from build123d import *

# Parameters (mm, degrees)
SKETCH_1_R          = 3.5
EXTRUDE_1_DEPTH     = 3
SKETCH_2_R          = 2
EXTRUDE_2_DEPTH     = 1
SKETCH_3_R          = 1.5
EXTRUDE_3_DEPTH     = 8
SKETCH_4_R          = 1
CUT_EXTRUDE_1_DEPTH = 1.5
FILLET_1_R          = 0.5
CHAMFER_1_SIZE      = 0.5


with BuildPart() as part:
    # 草图1 → 凸台-拉伸1 (new body)
    with BuildSketch(Plane(origin=(0, 0, 0), x_dir=(1, 0, 0), z_dir=(0, 1, 0))):
        with Locations(Location((0, 0, 0), (0, 0, 270))):
            Circle(SKETCH_1_R)
    extrude(amount=EXTRUDE_1_DEPTH)

    # 草图2 → 凸台-拉伸2 (add)
    with BuildSketch(Plane(origin=(0, 3, 0), x_dir=(1, 0, 0), z_dir=(0, 1, 0))):
        with Locations(Location((0, 0, 0), (0, 0, 270))):
            Circle(SKETCH_2_R)
    extrude(amount=EXTRUDE_2_DEPTH)

    # 草图3 → 凸台-拉伸3 (add)
    with BuildSketch(Plane(origin=(0, 4, 0), x_dir=(1, 0, 0), z_dir=(0, 1, 0))):
        with Locations(Location((0, 0, 0), (0, 0, 270))):
            Circle(SKETCH_3_R)
    extrude(amount=EXTRUDE_3_DEPTH)

    # 草图4 → 切除-拉伸1 (cut)
    with BuildSketch(Plane.XZ):
        with Locations(Location((0, 0, 0), (0, 0, 270))):
            Circle(SKETCH_4_R)
    extrude(amount=-CUT_EXTRUDE_1_DEPTH, mode=Mode.SUBTRACT)

    # 圆角1
    fillet_1_edges = [part.edges().sort_by_distance(p)[0] for p in [
        (0, 0, -3.5),
        (0, 3, -3.5),
    ]]
    fillet(fillet_1_edges, radius=FILLET_1_R)

    # 倒角1
    chamfer_1_edges = [part.edges().sort_by_distance(p)[0] for p in [
        (0, 12, -1.5),
    ]]
    chamfer(chamfer_1_edges, length=CHAMFER_1_SIZE)


solid = part.part
Input: part model. Units: mm. Frame: model coordinates. A direction names the side the tool comes from. Round coordinates to 2 decimals unless told otherwise and drop trailing zeros. Order: outer loops, then holes, each group sorted by start corner. A loop starts at its lowest first (then second) coordinate and runs counter-clockwise, first axis right, second up. Notation, with made-up numbers: (-25, -29) - (30, -29) arc R16 ccw to (30, -5) - close; hole circle Ø5 at (75.5, 56.5). An arc over 180 degrees is marked (long way). Use a Markdown table: item, result.
1. Section C-C on y = 6.5. Return the cut outline in (x, z).
Evaluation:
| item | result |
|---|---|
| outline | circle Ø3 at (0, 0) |
2. Section B-B on x = 0. Return the cut outline in (y, z).
Evaluation:
| item | result |
|---|---|
| outline | (0, -3) arc R0.5 ccw to (0.5, -3.5) - (2.5, -3.5) arc R0.5 ccw to (3, -3) - (3, -2) - (4, -2) - (4, -1.5) - (11.5, -1.5) - (12, -1) - (12, 1) - (11.5, 1.5) - (4, 1.5) - (4, 2) - (3, 2) - (3, 3) arc R0.5 ccw to (2.5, 3.5) - (0.5, 3.5) arc R0.5 ccw to (0, 3) - (0, 1) - (1.5, 1) - (1.5, -1) - (0, -1) - close |
3. Mould query, pull axis Z, two halves, no side actions, for faces 1 (the face through (0, 1.5, 0)), 2 (the face through (-1.952, 3.493, -0.434)), 3 (the face through (1, 0, -1)). Classes: +Z half, -Z half, draft (parallel to the pull), parting line (faces both ways), or undercut.
Evaluation:
| item | result |
|---|---|
| face 1 | undercut |
| face 2 | parting line |
| face 3 | draft |
4. Section A-A on z = 0. Return the cut outline in (x, y).
Evaluation:
| item | result |
|---|---|
| outline | (-3.5, 0.5) arc R0.5 ccw to (-3, 0) - (-1, 0) - (-1, 1.5) - (1, 1.5) - (1, 0) - (3, 0) arc R0.5 ccw to (3.5, 0.5) - (3.5, 2.5) arc R0.5 ccw to (3, 3) - (2, 3) - (2, 4) - (1.5, 4) - (1.5, 11.5) - (1, 12) - (-1, 12) - (-1.5, 11.5) - (-1.5, 4) - (-2, 4) - (-2, 3) - (-3, 3) arc R0.5 ccw to (-3.5, 2.5) - close |
5. Material intervals for probe 1 along X at (y, z) = (0.75, 0); probe 2 along Y at (x, z) = (0.75, -2); probe 3 along Y at (x, z) = (-1.75, 0), sorted ascending.
Evaluation:
| item | result |
|---|---|
| probe 1 | -3.5 to -1, 1 to 3.5 |
| probe 2 | 0 to 3 |
| probe 3 | 0 to 4 |
6. First-contact query: pin 1 (4 mm diameter, centred on x = 1, z = 0.5, fed in from -Y); pin 2 (3 mm diameter, centred on y = 9.5, z = 1.5, fed in from +X); pin 3 (1.5 mm diameter, centred on x = 0, y = 8.5, fed in from -Z); pin 4 (1 mm diameter, centred on x = -1.5, y = 7, fed in from +Z). Flat tips, straight axial feed; report the tip coordinate or a pass-through.
Evaluation:
| item | result |
|---|---|
| pin 1 | y = 0 |
| pin 2 | x = 1.5 |
| pin 3 | z = -1.5 |
| pin 4 | z = 1.12 |
7. Access query for faces 4 (the face through (-3.417, 1.486, -0.759)), 5 (the face through (-1, 1, 0)), 6 (the face through (-2, 3, 1)). Directions: +Z, -Z, +X, -X, +Y, -Y. A direction counts if a zero-diameter tool reaches every point of the face in a straight line with its end or side. Return the directions, or none.
Evaluation:
| item | result |
|---|---|
| face 4 | +Y, -Y |
| face 5 | -Y |
| face 6 | +Y |
